from build123d import *

# Parameters (mm, degrees)
BOSS_EXTRUDE1_DEPTH      = 0.405
FILLET1_R                = 1.12
CHAMFER1_SIZE            = 0.5
SKETCH2_R                = 1.1
CUT_EXTRUDE1_DEPTH       = 16.574075414
BOSS_EXTRUDE2_DEPTH      = 0.5
BOSS_EXTRUDE2_DEPTH_BACK = 5.1
SKETCH4_W                = 2.941717286
SKETCH4_H                = 0.549853698
BOSS_EXTRUDE3_DEPTH      = 0.05
BOSS_EXTRUDE4_DEPTH      = 0.525
SKETCH6_R                = 0.577649515
CUT_EXTRUDE2_DEPTH       = 17.26947218


with BuildPart() as part:
    # Sketch1 → Boss-Extrude1 (new, symmetric)
    with BuildSketch(Plane(origin=(0, 0, 0), x_dir=(1, 0, 0), z_dir=(0, 1, 0))):
        Polygon((-13.55, 7.635), (11.83, 7.635), (11.83, 3.675), (13.55, 2.295), (13.55, -2.295), (11.83, -3.675), (11.83, -7.635), (-13.55, -7.635), align=None)
    extrude(amount=BOSS_EXTRUDE1_DEPTH, both=True)

    # Fillet1
    fillet1_edges = [part.edges().sort_by_distance(p)[0] for p in [
        (-13.55, 0, -7.635),
        (-13.55, 0, 7.635),
    ]]
    fillet(fillet1_edges, radius=FILLET1_R)

    # Chamfer1
    chamfer1_edges = [part.edges().sort_by_distance(p)[0] for p in [
        (11.83, 0, -7.635),
        (11.83, 0, 7.635),
    ]]
    chamfer(chamfer1_edges, length=CHAMFER1_SIZE)

    # Sketch2 → Cut-Extrude1 (cut, through all)
    with BuildSketch(Plane(origin=(0, 0.405, 0), x_dir=(1, 0, 0), z_dir=(0, 1, 0))):
        with Locations(Location((9.57, 5.74, 0), (0, 0, 270))):
            Circle(SKETCH2_R)
        with Locations(Location((9.57, -5.74, 0), (0, 0, 270))):
            Circle(SKETCH2_R)
    extrude(amount=-CUT_EXTRUDE1_DEPTH, mode=Mode.SUBTRACT)

    # Sketch4 → Boss-Extrude3 (add)
    with BuildSketch(Plane(origin=(0, 0.405, 0), x_dir=(1, 0, 0), z_dir=(0, 1, 0))):
        with Locations((-10.930908088, 4.275112504)):
            Rectangle(SKETCH4_W, SKETCH4_H)
        with Locations((-10.930908088, -4.275112504)):
            Rectangle(SKETCH4_W, SKETCH4_H)
    extrude(amount=BOSS_EXTRUDE3_DEPTH)



with BuildPart() as body_2:
    # Sketch3 → Boss-Extrude2 (new, two sides: drawn at the far end of the back side and taken through both)
    with BuildSketch(Plane.ZY.offset(13.55).offset(-BOSS_EXTRUDE2_DEPTH_BACK)):
        Polygon((-3.91, 1.655), (-2.42, 0.455), (2.42, 0.455), (3.91, 1.655), (3.91, 2.505), (2.42, 3.405), (-2.42, 3.405), (-3.91, 2.505), align=None)
    extrude(amount=BOSS_EXTRUDE2_DEPTH + BOSS_EXTRUDE2_DEPTH_BACK)


with BuildPart() as part_1:
    add(part.part)

    add(body_2.part)  # Boss-Extrude4 merges body 2
    # Sketch5 → Boss-Extrude4 (add, symmetric)
    with BuildSketch(Plane(origin=(-11, 0, 0), x_dir=(0, 0, -1), z_dir=(1, 0, 0))):
        Polygon((4.325381098, 0.455), (4.325381098, 0.509426612), (4.162105788, 0.509426612), (3.964358919, 1.644096311), (3.498388432, 1.644096311), (3.498388432, 1.44259556), (3.964358919, 1.44259556), (4.136474144, 0.455), align=None)
        Polygon((-4.136474144, 0.455), (-4.325381098, 0.455), (-4.325381098, 0.509426612), (-4.162105788, 0.509426612), (-3.964358919, 1.644096311), (-3.498388432, 1.644096311), (-3.498388432, 1.44259556), (-3.964358919, 1.44259556), align=None)
    extrude(amount=BOSS_EXTRUDE4_DEPTH, both=True)

    # Sketch6 → Cut-Extrude2 (cut, through all)
    with BuildSketch(Plane(origin=(0, 0.405, 0), x_dir=(1, 0, 0), z_dir=(0, 1, 0))):
        with Locations(Location((-5.985172419, 5.913658107, 0), (0, 0, 270))):
            Circle(SKETCH6_R)
        with Locations(Location((-3.485172419, 5.913658107, 0), (0, 0, 270))):
            Circle(SKETCH6_R)
        with Locations(Location((-0.985172419, 5.913658107, 0), (0, 0, 270))):
            Circle(SKETCH6_R)
        with Locations(Location((1.514827581, 5.913658107, 0), (0, 0, 270))):
            Circle(SKETCH6_R)
        with Locations(Location((4.014827581, 5.913658107, 0), (0, 0, 270))):
            Circle(SKETCH6_R)
        with Locations(Location((4.014827581, -5.913658107, 0), (0, 0, 90))):
            Circle(SKETCH6_R)
        with Locations(Location((1.514827581, -5.913658107, 0), (0, 0, 90))):
            Circle(SKETCH6_R)
        with Locations(Location((-0.985172419, -5.913658107, 0), (0, 0, 90))):
            Circle(SKETCH6_R)
        with Locations(Location((-3.485172419, -5.913658107, 0), (0, 0, 90))):
            Circle(SKETCH6_R)
        with Locations(Location((-5.985172419, -5.913658107, 0), (0, 0, 90))):
            Circle(SKETCH6_R)
    extrude(amount=-CUT_EXTRUDE2_DEPTH, mode=Mode.SUBTRACT)


solid = part_1.part
Check sheet for the modelled part. Datum: model origin and axes. Units: mm. A direction names the side the tool comes from. Round coordinates to 2 decimals unless told otherwise and drop trailing zeros. Order: outer loops, then holes, each group sorted by start corner. A loop starts at its lowest first (then second) coordinate and runs counter-clockwise, first axis right, second up. Notation, with made-up numbers: M 51,20.25 L 106,20.25 A22 ccw 106,28.25 Z; hole C -39.5,82 d8. An arc over 180 degrees is marked long. One line per item, written item: value. Start each with the question number.
1. Section check D-D on z = -5.74. Enter the section's corners in (x, y) (3 decimals), and give its area (3 significant figures).
2. Section check A-A on x = 9.57. Enter the section's corners in (y, z) (3 decimals).
3. Gauge pin test, flat ends, axial feed: P1, Ø1, axis at y = 1, z = -3, coming from the +X side; P2, Ø6, axis at x = -1, z = -3.5, coming from the +Y side (3 decimals); P3, Ø1, axis at x = 1.51, z = 5.91, coming from the -Y side; P4, Ø0.9, axis at x = -11.5, y = 2, coming from the +Z side. Record the tip position at first contact, or that the pin passes through.
4. Scan lines: line 1 along Y through (x, z) = (-2, -1) (3 decimals); line 2 along Z through (x, y) = (4.5, 0) (3 decimals); line 3 along X through (y, z) = (1.25, -0.5). Record each from-to range of solid material in increasing order.
5. Release check for a two-part mould opening along Z. For faces 1 (the flat face through (-8.45, 2, 0)), 2 (the flat face through (12.678, 0.006, -2.995)), 3 (the cylindrical face through (-13.21, 0.01, 7.32)), 4 (the flat face through (-11.211, 1.047, 3.155)) record: released by +Z, released by -Z, zero draft, split by the parting line, or undercut.
6. Section check C-C on y = 2.2. Enter the section's corners in (x, z).
7. Section check B-B on z = 0.5. Enter the section's corners in (x, y) (3 decimals).
8. Access from +Z, -Z, +X, -X, +Y, -Y to the whole of each face (thin tool, end or side, straight path). Record for faces 5 (the flat face through (-11, 2, 3.91)), 6 (the flat face through (-13.55, 0, 0)), 7 (the cylindrical face through (-0.96, 0.01, -6.49)), 8 (the flat face through (11.83, 0, 5)).
Results found:
1. outline: M -13.55,-0.405 L -6.536,-0.405 L -6.536,0.405 L -13.55,0.405 Z; M -5.434,-0.405 L -4.036,-0.405 L -4.036,0.405 L -5.434,0.405 Z; M -2.934,-0.405 L -1.536,-0.405 L -1.536,0.405 L -2.934,0.405 Z; M -0.434,-0.405 L 0.964,-0.405 L 0.964,0.405 L -0.434,0.405 Z; M 2.066,-0.405 L 3.464,-0.405 L 3.464,0.405 L 2.066,0.405 Z; M 4.566,-0.405 L 8.47,-0.405 L 8.47,0.405 L 4.566,0.405 Z; M 10.67,-0.405 L 11.83,-0.405 L 11.83,0.405 L 10.67,0.405 Z
1. area: 14.3 mm^2
2. outline: M -0.405,-7.635 L 0.405,-7.635 L 0.405,-6.84 L -0.405,-6.84 Z; M -0.405,-4.64 L 0.405,-4.64 L 0.405,4.64 L -0.405,4.64 Z; M -0.405,6.84 L 0.405,6.84 L 0.405,7.635 L -0.405,7.635 Z
3. P1: x = -8.45
3. P2: y = 0.405
3. P3: through
3. P4: z = 3.98
4. line 1: -0.405 to 0.405
4. line 2: -7.635 to -6.227, -5.6 to 5.6, 6.227 to 7.635
4. line 3: -14.05 to -8.45
5. face 1: zero draft
5. face 2: released by -Z
5. face 3: released by +Z
5. face 4: undercut
6. outline: M -14.05,-3.91 L -8.45,-3.91 L -8.45,3.91 L -14.05,3.91 Z
7. outline: M -14.05,0.455 L -8.45,0.455 L -8.45,3.405 L -14.05,3.405 Z; M -13.55,-0.405 L 13.55,-0.405 L 13.55,0.405 L -13.55,0.405 Z
8. face 5: +Z, +X, -X, +Y
8. face 6: +Z, -Z, -X, -Y
8. face 7: +Y, -Y
8. face 8: +Z, +X, +Y, -Y
